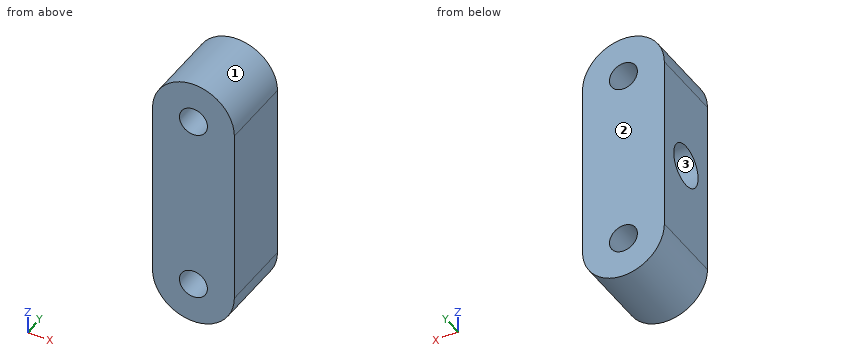
```python
from build123d import *

# Parameters (mm, degrees)
EXTRUDE_1_DEPTH     = 11
SKETCH_2_R          = 2.05
CUT_EXTRUDE_1_DEPTH = 12
SKETCH_3_R          = 3.1
CUT_EXTRUDE_2_DEPTH = 10


with BuildPart() as part:
    # 草图1 → 凸台-拉伸1 (new body)
    with BuildSketch(Plane(origin=(0, 0, 0), x_dir=(1, 0, 0), z_dir=(0, 1, 0))):
        with BuildLine():
            Line((-6, -13), (-6, 13))
            ThreePointArc((-6, 13), (0, 19), (6, 13))
            Line((6, 13), (6, -13))
            ThreePointArc((6, -13), (0, -19), (-6, -13))
        make_face()
    extrude(amount=EXTRUDE_1_DEPTH)

    # 草图2 → 切除-拉伸1 (cut, through all)
    with BuildSketch(Plane(origin=(0, 11, 0), x_dir=(1, 0, 0), z_dir=(0, 1, 0))):
        with Locations((0, 13)):
            Circle(SKETCH_2_R)
        with Locations((0, -13)):
            Circle(SKETCH_2_R)
    extrude(amount=-CUT_EXTRUDE_1_DEPTH, mode=Mode.SUBTRACT)

    # 草图3 → 切除-拉伸2 (cut)
    with BuildSketch(Plane.ZY.offset(6)):
        with Locations((0, 5.5)):
            Circle(SKETCH_3_R)
    extrude(amount=-CUT_EXTRUDE_2_DEPTH, mode=Mode.SUBTRACT)


solid = part.part
```
CAD build for the part. Positions are in the model's coordinates, mm. Face numbers are marked on the shaded views. Coordinates: 2 decimals unless noted, no trailing zeros. Loops run counter-clockwise (first coordinate to the right, second up) from the corner with the lowest first, then second, coordinate; pieces in that order, holes last. Notation, with made-up numbers: (62.5, 73) - (115.5, 73) arc R17 cw to (115.5, 94) - close; hole circle Ø11 at (32.5, 48). An arc over 180 degrees is marked (long way). Return JSON: item names as keys, results as strings.
1. Probe L1, parallel to Y at x = 0.5, z = 0; L2, parallel to X at y = 6.5, z = 13; L3, parallel to Z at x = 0, y = 7.5. List the from-to ranges inside material, lowest first. Write a range as from..to.
Result:
{"L1": "y = 0..2.4, 8.6..11", "L2": "x = -6..-2.05, 2.05..6", "L3": "z = -19..-15.05, -10.95..-2.37, 2.37..10.95, 15.05..19"}
2. Band-saw the part on B-B (y = 5.5). Give the cut face in (x, z), and give its area (3 significant figures).
Result:
{"outline": "(-6, -13) arc R6 ccw to (6, -13) - (6, 13) arc R6 ccw to (-6, 13) - (-6, 3.1) - (4, 3.1) - (4, -3.1) - (-6, -3.1) - close; hole circle Ø4.1 at (0, -13); hole circle Ø4.1 at (0, 13)", "area": "337 mm2"}
3. Band-saw the part on A-A (x = 0). Give the cut face in (y, z).
Result:
{"outline": "(0, -19) - (11, -19) - (11, -15.05) - (0, -15.05) - close; (0, -10.95) - (11, -10.95) - (11, 10.95) - (0, 10.95) - close; (0, 15.05) - (11, 15.05) - (11, 19) - (0, 19) - close; hole circle Ø6.2 at (5.5, 0)"}
4. Band-saw the part on C-C (z = 0). Give the cut face in (x, y), and give its area (3 significant figures).
Result:
{"outline": "(-6, 0) - (6, 0) - (6, 11) - (-6, 11) - (-6, 8.6) - (4, 8.6) - (4, 2.4) - (-6, 2.4) - close", "area": "70.0 mm2"}
5. Band-saw the part on D-D (x = -3.25). Give the cut face in (y, z), and give its area (3 significant figures).
Result:
{"outline": "(0, -18.04) - (11, -18.04) - (11, 18.04) - (0, 18.04) - close; hole circle Ø6.2 at (5.5, 0)", "area": "367 mm2"}
6. Drop flat-ended pins along their axis: pin 1 (3 mm diameter, centred on x = -3, y = 8.5, fed in from +Z); pin 2 (1 mm diameter, centred on y = 6.5, z = 13.5, fed in from +X); pin 3 (1 mm diameter, centred on x = -3, y = 1.5, fed in from +Z); pin 4 (5 mm diameter, centred on y = 5.5, z = 0, fed in from -X). Give the stop position or say it passes through.
Result:
{"pin 1": "stops at z = 18.81", "pin 2": "stops at x = 6", "pin 3": "stops at z = 18.45", "pin 4": "stops at x = 4"}
7. Mould opens along Z. For the marked faces 1, 2 and 3 say: released by +Z, released by -Z, zero draft, split by the parting line, or undercut.
Result:
{"face 1": "released by +Z", "face 2": "zero draft", "face 3": "undercut"}
